For this review, take the finished solid that the model builds, in its own axes (mm). A direction names the side the tool comes from. Coordinates: 2 decimals unless noted, no trailing zeros. Write each loop counter-clockwise with the first axis right and the second up, starting at its lowest first coordinate (ties: lowest second). Pieces come first, ordered by that corner, then holes.
Solid Edge part; units mm, degrees
sketch "Sketch1" plane through (0, 0, 0) normal (0, -1, 0) x (1, 0, 0)
  line L0 (-92.8835, -54.8099) -> (-82.8835, -54.8099)
  line L1 (-82.8835, -54.8099) -> (-82.8835, 45.1901)
  line L2 (-82.8835, 45.1901) -> (-92.8835, 45.1901)
  line L3 (-92.8835, 45.1901) -> (-92.8835, -54.8099)
  dimension "D1" = 82.8835
  dimension "D2" = 92.8835
extrude "Protrusion1" add sketch "Sketch1" against normal blind 208
sketch "Sketch2" plane through (-82.8835, 104, 0.1901) normal (1, 0, 0) x (0, -1, 0)
  line L0 (-50, -35) -> (50, -35)
  line L1 (50, -35) -> (50, 55)
  line L2 (50, 55) -> (-50, 55)
  line L3 (-50, 55) -> (-50, -35)
  dimension "D1" = 50
  dimension "D2" = 50
extrude "Protrusion2" add sketch "Sketch2" along normal blind 20
sketch "Sketch3" plane through (-82.8835, 100, 10.1901) normal (1, 0, 0) x (0, -1, 0)
  circle A0 centre (58.5, -10) radius 5
  circle A1 centre (-66.5, -10) radius 5
extrude "Cutout1" cut sketch "Sketch3" against normal through all
extrude "ExtrudedCutout_6" [suppressed]
sketch "Sketch4" plane through (-92.8835, 145.5, -4.8099) normal (-1, 0, 0) x (0, 1, 0)
  circle A0 centre (-18.5, 35) radius 3
  circle A1 centre (-18.5, -11) radius 3
  circle A2 centre (-64.5, -11) radius 3
  circle A3 centre (-64.5, 35) radius 3
extrude "Cutout2" cut sketch "Sketch4" against normal through all
sketch "Sketch5" plane through (-92.8835, 145.5, 0.1901) normal (-1, 0, 0) x (0, -1, 0)
  circle A0 centre (18.5, -40) radius 5
  circle A1 centre (64.5, -40) radius 5
  circle A2 centre (64.5, 6) radius 5
  circle A3 centre (18.5, 6) radius 5
extrude "Cutout3" cut sketch "Sketch5" against normal up to vertex (40 mm away)
sketch "Sketch6" plane through (-92.8835, 104, -4.8099) normal (-1, 0, 0) x (0, -1, 0)
  circle A0 centre (62.5, 25) radius 15
  circle A1 centre (-62.5, 25) radius 10
  circle A2 centre (62.5, 25) radius 10
  circle A3 centre (-62.5, 25) radius 15
extrude "ExtrudedCutout_9" cut sketch "Sketch6" against normal blind 2
properties material "Aluminum, 6061-T6"
Q1. Add section C-C (z = -42). State the section outline as (x, y) points, then the cut area to 3 significant figures.
Ans:
outline: (-92.88, 0) - (-82.88, 0) - (-82.88, 54) - (-62.88, 54) - (-62.88, 76.51) - (-92.88, 76.51) - close; (-92.88, 85.49) - (-62.88, 85.49) - (-62.88, 122.51) - (-92.88, 122.51) - close; (-92.88, 131.49) - (-62.88, 131.49) - (-62.88, 154) - (-82.88, 154) - (-82.88, 208) - (-92.88, 208) - close
area: 3,540 mm2
Q2. Add section D-D (x = -84.75). State the section outline as (y, z) points.
Ans:
outline: (0, -54.81) - (208, -54.81) - (208, 45.19) - (0, 45.19) - close; hole circle Ø10 at (41.5, 20.19); hole circle Ø10 at (81, -39.81); hole circle Ø10 at (81, 6.19); hole circle Ø10 at (127, -39.81); hole circle Ø10 at (127, 6.19); hole circle Ø10 at (166.5, 20.19)
Q3. For probe 1 along Z at (x, y) = (-92.2, 41.5); probe 2 along Z at (x, y) = (-76, 81); probe 3 along Z at (x, y) = (-86.5, 127), list the stretches that pass through material, from the lowest coordinate up.
Ans:
probe 1: z = -54.81 to 5.19, 10.19 to 15.19, 25.19 to 30.19, 35.19 to 45.19
probe 2: z = -54.81 to -44.81, -34.81 to 1.19, 11.19 to 35.19
probe 3: z = -54.81 to -44.81, -34.81 to 1.19, 11.19 to 45.19
Q4. Draft analysis for pull direction Y (two halves, no side actions). For faces 6 (the flat face through (-88, 103, 45.19)), 7 (the flat face through (-73, 154, -10)), 8 (the cylindrical face through (-78.09, 122.38, -41.72)), 9 (the flat face through (-88, 0, -4)), state which applies: +Y half, -Y half, draft (parallel to the pull), parting line (faces both ways), or undercut.
Ans:
face 6: draft
face 7: +Y half
face 8: undercut
face 9: -Y half
Q5. Clearance check with flat-ended pins moving along their axes: pin 1 Ø16 at (y, z) = (41.5, 20.19) entering from +X; pin 2 Ø16 at (y, z) = (81, 6.19) entering from +X; pin 3 Ø1.5 at (x, z) = (-69.5, 11.5) entering from +Y; pin 4 Ø10 at (x, y) = (-75, 124.5) entering from +Z. State where each tip first meets the part, or that it passes through.
Ans:
pin 1: stops at x = -82.88
pin 2: stops at x = -62.88
pin 3: stops at y = 154
pin 4: stops at z = 35.19
Q6. Add section A-A (y = 127). State the section outline as (x, z) points.
Ans:
outline: (-92.88, -54.81) - (-62.88, -54.81) - (-62.88, -44.81) - (-92.88, -44.81) - close; (-92.88, -34.81) - (-62.88, -34.81) - (-62.88, 1.19) - (-92.88, 1.19) - close; (-92.88, 11.19) - (-62.88, 11.19) - (-62.88, 35.19) - (-82.88, 35.19) - (-82.88, 45.19) - (-92.88, 45.19) - close
Q7. Tool access review of faces 1 (the cylindrical face through (-78.09, 76.38, 4.28)), 2 (the flat face through (-73, 54, -9)), 3 (the flat face through (-82.884, 103, 39)), 4 (the cylindrical face through (-91.898, 56.485, 20.85)), 5 (the flat face through (-62.884, 103, -10)): name each direction out of +Z, -Z, +X, -X, +Y, -Y from which nothing blocks a thin tool from reaching the whole face with its end or side.
Ans:
face 1: +X, -X
face 2: +Z, -Z, +X, -Y
face 3: +Z, +X
face 4: -X
face 5: +Z, -Z, +X, +Y, -Y
Q8. Add section B-B (y = 41.5). State the section outline as (x, z) points, then the cut area to 3 significant figures.
Ans:
outline: (-92.88, -54.81) - (-82.88, -54.81) - (-82.88, 15.19) - (-92.88, 15.19) - (-92.88, 10.19) - (-90.88, 10.19) - (-90.88, 5.19) - (-92.88, 5.19) - close; (-92.88, 25.19) - (-82.88, 25.19) - (-82.88, 45.19) - (-92.88, 45.19) - (-92.88, 35.19) - (-90.88, 35.19) - (-90.88, 30.19) - (-92.88, 30.19) - close
area: 880 mm2
